Source: CAD feature listing. Evaluate the final solid. Frame: model axes, mm. A direction names the side the tool comes from. Give positions to 0.01 mm unless a question says otherwise; leave off trailing zeros. Order: outer loops, then holes, each group sorted by start corner. A loop starts at its lowest first (then second) coordinate and runs counter-clockwise, first axis right, second up. Notation, with made-up numbers: (26, 66) - (52, 66) arc R25 cw to (52, 100) - close; hole circle Ø3 at (-32, 34.25). An arc over 180 degrees is marked (long way). Write each question's results on one line, items separated by ' | '. Start each with the question number.
Item 1: Section B-B on x = -28. Output: boundary loops of the cut face in (y, z), and give its area (3 significant figures).
Item 2: Contact query for flat-ended pins moving along their axis: pin 1 Ø10 at (y, z) = (61, 37.5) entering from +X; pin 2 Ø3 at (x, y) = (36.5, 53.5) entering from +Z; pin 3 Ø6.5 at (y, z) = (42, 4.5) entering from +X. Output: stop coordinate, or through.
Item 3: Mould query, pull axis Z, two halves, no side actions, for faces 1 (the flat face through (32, 38, 25.4)), 2 (the flat face through (-32, 38, 38.1)), 3 (the flat face through (-88.9, 38, 26)). Classes: released by +Z, released by -Z, zero draft, split by the parting line, or undercut.
Item 4: Set-up query: faces 4 (the flat face through (-31, 76.2, 20)), 5 (the flat face through (-63.5, 38, 44)), 6 (the flat face through (0, 38, 8)), 7 (the flat face through (-70, 38, 38.1)). Return all of +Z, -Z, +X, -X, +Y, -Y with unobstructed straight access to the full face (end or side cutting, diameter ignored); none if empty.
Item 5: Line query: line 1 along Z through (x, y) = (-29, 13); line 2 along Z through (x, y) = (-61.5, 52); line 3 along Z through (x, y) = (49, 31.5). Output: solid intervals per line, ascending.
Item 6: Section D-D on x = 43. Output: boundary loops of the cut face in (y, z).
Item 7: Section C-C on y = 44.5. Output: boundary loops of the cut face in (x, z).
Item 8: Section A-A on z = 43. Output: boundary loops of the cut face in (x, y).
```python
from build123d import *

# Parameters (mm, degrees)
F1_DEPTH = 76.2
F3_DEPTH = 203.2


with BuildPart() as f1:
    # F0 (on Front) → F1 (new body)
    with BuildSketch(Plane.XZ):
        Polygon((-88.9, 50.8), (-88.9, 0), (63.5, 0), (63.5, 25.4), (0, 25.4), (-12.7, 50.8), (-38.1, 50.8), (-38.1, 38.1), (-25.4, 38.1), (-25.4, 25.4), (-76.2, 25.4), (-76.2, 38.1), (-63.5, 38.1), (-63.5, 50.8), align=None)
    extrude(amount=-F1_DEPTH)

    # F2 (on Right) → F3 (cut)
    with BuildSketch(Plane.YZ):
        Polygon((63.425437, 12.6984), (12.625437, 12.6984), (25.4, 0), (50.8, 0), align=None)
    extrude(amount=F3_DEPTH, mode=Mode.SUBTRACT)


solid = f1.part
```
Evaluation:
1) outline: (0, 0) - (76.2, 0) - (76.2, 25.4) - (0, 25.4) - close; (0, 38.1) - (76.2, 38.1) - (76.2, 50.8) - (0, 50.8) - close | area: 2,900 mm^2
2) pin 1: stops at x = -3.55 | pin 2: stops at z = 25.4 | pin 3: stops at x = 0
3) face 1: released by +Z | face 2: undercut | face 3: zero draft
4) face 4: +Z, -Z, +X, -X, +Y | face 5: +Z, +Y, -Y | face 6: +X | face 7: +Y, -Y
5) line 1: z = 0 to 25.4, 38.1 to 50.8 | line 2: z = 0 to 25.4 | line 3: z = 12.7 to 25.4
6) outline: (0, 0) - (25.4, 0) - (12.63, 12.7) - (63.43, 12.7) - (50.8, 0) - (76.2, 0) - (76.2, 25.4) - (0, 25.4) - close
7) outline: (-88.9, 0) - (0, 0) - (0, 12.7) - (63.5, 12.7) - (63.5, 25.4) - (0, 25.4) - (-12.7, 50.8) - (-38.1, 50.8) - (-38.1, 38.1) - (-25.4, 38.1) - (-25.4, 25.4) - (-76.2, 25.4) - (-76.2, 38.1) - (-63.5, 38.1) - (-63.5, 50.8) - (-88.9, 50.8) - close
8) outline: (-88.9, 0) - (-63.5, 0) - (-63.5, 76.2) - (-88.9, 76.2) - close; (-38.1, 0) - (-8.8, 0) - (-8.8, 76.2) - (-38.1, 76.2) - close
